from build123d import *

# Parameters (mm, degrees)
BOSS_EXTRUDE1_DEPTH = 3
SKETCH2_R           = 1.5
CUT_EXTRUDE1_DEPTH  = 19.275667036
SKETCH3_W           = 10
SKETCH3_H           = 120
BOSS_EXTRUDE2_DEPTH = 3


with BuildPart() as part:
    # Sketch1 → Boss-Extrude1 (new body)
    with BuildSketch(Plane(origin=(0, 0, 0), x_dir=(1, 0, 0), z_dir=(0, 1, 0))):
        with BuildLine():
            Line((0, 0), (10, 0))
            add(Edge.make_bspline(
                [(10, 0), (10, 15), (5, 15), (0, 15), (0, 0)],
                knots=[4.71238898, 4.71238898, 4.71238898, 6.283185307, 6.283185307, 7.853981634, 7.853981634, 7.853981634], degree=2, weights=[1, 0.707106781, 1, 0.707106781, 1]))
        make_face()
    boss_extrude1 = extrude(amount=BOSS_EXTRUDE1_DEPTH)

    # Sketch2 → Cut-Extrude1 (cut, through all)
    with BuildSketch(Plane(origin=(0, 3, 0), x_dir=(1, 0, 0), z_dir=(0, 1, 0))):
        with Locations(Location((5, 9, 0), (0, 0, 270))):
            Circle(SKETCH2_R)
    cut_extrude1 = extrude(amount=-CUT_EXTRUDE1_DEPTH, mode=Mode.SUBTRACT)

    # Sketch3 → Boss-Extrude2 (add)
    with BuildSketch(Plane.XY):
        with Locations((5, -57)):
            Rectangle(SKETCH3_W, SKETCH3_H)
    extrude(amount=-BOSS_EXTRUDE2_DEPTH)

    # Mirror1: Boss-Extrude1, Cut-Extrude1 across plane
    add(boss_extrude1.mirror(Plane.ZX.offset(-57)))
    add(cut_extrude1.mirror(Plane.ZX.offset(-57)), mode=Mode.SUBTRACT)


solid = part.part
Geometry: final body of the model. Coordinates: model frame, mm. A direction names the side the tool comes from. Give positions to 0.01 mm unless a question says otherwise; leave off trailing zeros. Write each loop counter-clockwise with the first axis right and the second up, starting at its lowest first coordinate (ties: lowest second). Pieces come first, ordered by that corner, then holes.
(1) Access query for faces 5 (the flat face through (5, -117, -6)), 6 (the flat face through (3.8, 0, -7.8)). Directions: +Z, -Z, +X, -X, +Y, -Y. A direction counts if a zero-diameter tool reaches every point of the face in a straight line with its end or side. Return the directions, or none.
(2) First-contact query: P1, Ø6, axis at x = 4, y = -97.5, coming from the -Z side. Flat tip, straight axial feed; report the tip coordinate or a pass-through.
(3) Mould query, pull axis Z, two halves, no side actions, for faces 1 (the flat face through (0, -58, -1)), 2 (the flat face through (5, -56, -3)), 3 (the cylindrical face through (5.07, -115.52, -10.5)), 4 (the cylindrical face through (5.07, 1.52, -10.5)). Classes: released by +Z, released by -Z, zero draft, split by the parting line, or undercut.
(4) Ray query, line 1 (Y direction, x = 3, z = -12.25); line 2 (Z direction, x = 5, y = -114.8); line 3 (Z direction, x = 6.5, y = -17). Return the intervals inside material, ascending.
(5) Cut plane C-C, the plane y = -70. Return loops of the section in (x, z).
(6) Cut plane A-A, the plane z = -9. Give the number of separate pieces and of enclosed holes in the cut face, then the cut area to 3 significant figures.
Values follow:
1. face 5: +Z, -Z, +X, -X, -Y
1. face 6: -Z, +X, -X
2. P1: stops at z = -3
3. face 1: zero draft
3. face 2: released by -Z
3. face 3: undercut
3. face 4: undercut
4. line 1: y = -117 to -114, 0 to 3
4. line 2: z = -15 to -10.5, -7.5 to 0
4. line 3: z = -3 to 0
5. outline: (0, -3) - (10, -3) - (10, 0) - (0, 0) - close
6. separate pieces: 4
6. enclosed holes: 0
6. area: 30.0 mm2
